Build history of the part. All positions in model axes, mm. A direction names the side the tool comes from. Coordinates: 2 decimals unless noted, no trailing zeros. Order: outer loops, then holes, each group sorted by start corner. A loop starts at its lowest first (then second) coordinate and runs counter-clockwise, first axis right, second up. Notation, with made-up numbers: (25.5, -33) - (45.5, -33) arc R19 ccw to (45.5, -12) - close; hole circle Ø1 at (36.5, 24.5). An arc over 180 degrees is marked (long way). Write each question's results on one line, items separated by ' | '. Start each with the question number.
from build123d import *

# Parameters (mm, degrees)
PAD011_DEPTH              = 0.4
CHAMFER001_SIZE2          = 0.7
CHAMFER001_SIZE           = 0.1
SKETCH012_W               = 0.9
SKETCH012_H               = 0.85
PAD012_DEPTH              = 3
PAD010_DEPTH              = 4.2
CHAMFER_SIZE2             = 0.4
CHAMFER_SIZE              = 0.2
FUSION001_PLACEMENT_ANGLE = 180


with BuildPart() as chamfer001:
    # Sketch011 → Pad011 (new body)
    with BuildSketch(Plane.XY.offset(0.9)):
        Polygon((-7.65, 0), (7.65, 0), (7.65, -0.7), (7.4, -1.4), (-7.4, -1.4), (-7.65, -0.7), align=None)
    extrude(amount=PAD011_DEPTH)

    # Chamfer001
    chamfer001_edges = [chamfer001.edges().sort_by_distance(p)[0] for p in [
        (0, -1.4, 0.9),
    ]]
    chamfer001_side = chamfer001.faces().sort_by_distance((0, -1.4, 1.1))[0]
    chamfer(chamfer001_edges, length=CHAMFER001_SIZE, length2=CHAMFER001_SIZE2, reference=chamfer001_side)


with BuildPart() as body012:
    # Sketch012 → Pad012 (new body)
    with BuildSketch(Plane.XZ):
        Polygon((-10.325, 0), (-10.325, 1.8), (10.325, 1.8), (10.325, 0), (7.825, 0), (7.825, 0.9), (-7.825, 0.9), (-7.825, 0), align=None)
        with Locations((-9.025, 0.9)):
            Rectangle(SKETCH012_W, SKETCH012_H, mode=Mode.SUBTRACT)
        with Locations((9.025, 0.9)):
            Rectangle(SKETCH012_W, SKETCH012_H, mode=Mode.SUBTRACT)
    extrude(amount=PAD012_DEPTH)


with BuildPart() as fusion001:
    # Sketch010 → Pad010 (new body)
    with BuildSketch(Plane.XZ.offset(-1.3)):
        Polygon((-10.325, 0), (-10.325, 1.8), (10.325, 1.8), (10.325, 0), (7.825, 0), (7.825, 0.9), (-7.825, 0.9), (-7.825, 0), align=None)
    extrude(amount=PAD010_DEPTH)

    # Cut002: cut Body012
    add(body012.part, mode=Mode.SUBTRACT)

    # Chamfer
    chamfer_edges = [fusion001.edges().sort_by_distance(p)[0] for p in [
        (8.575, 0, 0.9),
        (9.025, 0, 0.475),
        (9.025, 0, 1.325),
        (-9.025, 0, 0.475),
        (-9.025, 0, 1.325),
        (-8.575, 0, 0.9),
    ]]
    chamfer_side = fusion001.faces().sort_by_distance((0, 0, 1.19405))[0]
    chamfer(chamfer_edges, length=CHAMFER_SIZE, length2=CHAMFER_SIZE2, reference=chamfer_side)

    # Fusion001: union Chamfer001
    add(chamfer001.part)


with BuildPart() as fusion001_1:
    # Fusion001 placement: moved
    add(fusion001.part.moved(Location((0, 1.1, 2))).rotate(Axis((0, 1.1, 2), (0, 1, 0)), FUSION001_PLACEMENT_ANGLE))


solid = fusion001_1.part
Item 1: Which spindle directions (+Z, -Z, +X, -X, +Y, -Y) get a long thin tool onto all of the face, cutting with end or side? Do faces 1 (the flat face through (9.475, 0, 1)), 2 (the flat face through (-8.575, -1, 1)), 3 (the flat face through (9, -1, 1.525)), 4 (the flat face through (7.825, 1.8, 1.5)). Say none if no direction does.
Item 2: Slice it at A-A (y = -1). Write the cut outline in (x, z) (3 decimals).
Item 3: Flat gauge pins, fed straight in: P1, Ø0.9, axis at y = 0, z = 1, coming from the -X side (3 decimals); P2, Ø0.7, axis at x = 9, y = -1, coming from the +Z side (3 decimals); P3, Ø2, axis at x = 2.5, y = 1.5, coming from the +Z side. Where does each tip first touch, or does it go through?
Item 4: Slice it at D-D (x = 9). Write the cut outline in (y, z) (3 decimals), then the cut area to 4 significant figures.
Item 5: Pull direction X, two halves, no side cores. Call faces 5 (the flat face through (-9, -1.8, 1)), 6 (the flat face through (-7.825, 1.8, 1.6)), 7 (the flat face through (8.575, -1, 1)), 8 (the flat face through (-10.325, 2, 1)): released by +X, released by -X, zero draft, split by the parting line, or undercut.
Item 6: Slice it at B-B (z = 1.35). Write the cut outline in (x, y) (3 decimals).
Item 7: Slice it at C-C (y = 1.65). Write the cut outline in (x, z) (3 decimals), then the cut area to 3 significant figures.
Item 8: Probe probe 1 along X at (y, z) = (0.45, 0.85) (3 decimals); probe 2 along X at (y, z) = (2.15, 1.25) (3 decimals); probe 3 along X at (y, z) = (0.95, 0.8) (3 decimals). List the from-to ranges inside material, lowest first.
Resolved:
1) face 1: +Z, -Z, +X, -Y | face 2: +Z, -Z, -Y | face 3: +Z, +X, -X, -Y | face 4: +Z, +Y, -Y
2) outline: (-9.475, 0.675) - (-8.575, 0.675) - (-8.575, 1.525) - (-9.475, 1.525) - close; (8.575, 0.675) - (9.475, 0.675) - (9.475, 1.525) - (8.575, 1.525) - close
3) P1: x = -9.475 | P2: z = 1.525 | P3: z = 1.1
4) outline: (-1.8, 0.675) - (0.7, 0.675) - (1.1, 0.475) - (1.1, 0.2) - (2.4, 0.2) - (2.4, 2) - (1.1, 2) - (1.1, 1.725) - (0.7, 1.525) - (-1.8, 1.525) - close | area: 4.885 mm^2
5) face 5: zero draft | face 6: undercut | face 7: undercut | face 8: released by -X
6) outline: (-10.325, 1.1) - (-9.475, 1.1) - (-9.475, -1.8) - (-8.575, -1.8) - (-8.575, 0.7) - (-8.375, 1.1) - (-7.825, 1.1) - (-7.825, 2.4) - (-10.325, 2.4) - close; (7.825, 1.1) - (8.375, 1.1) - (8.575, 0.7) - (8.575, -1.8) - (9.475, -1.8) - (9.475, 1.1) - (10.325, 1.1) - (10.325, 2.4) - (7.825, 2.4) - close
7) outline: (-10.325, 0.2) - (10.325, 0.2) - (10.325, 2) - (7.825, 2) - (7.825, 1.1) - (-7.825, 1.1) - (-7.825, 2) - (-10.325, 2) - close | area: 23.1 mm^2
8) probe 1: -9.475 to -8.575, -7.65 to 7.65, 8.575 to 9.475 | probe 2: -10.325 to -7.825, 7.825 to 10.325 | probe 3: -9.475 to -8.45, -7.65 to 7.65, 8.45 to 9.475
